Autodesk Inventor part; units mm, degrees
ref_plane "YZ Plane" through (0, 0, 0) normal (1, 0, 0) x (0, 1, 0)
ref_plane "XZ Plane" through (0, 0, 0) normal (0, 1, 0) x (-1, 0, 0)
ref_plane "XY Plane" through (0, 0, 0) normal (0, 0, 1) x (1, 0, 0)
sketch "Sketch1" plane through (0, 0, 0) normal (0, 0, 1) x (1, 0, 0)
  line L0 (0, 6) -> (0, 9)
  line L1 (0, 9) -> (10, 9)
  line L2 (10, 9) -> (10, 0)
  line L3 (10, 0) -> (0, 0)
  line L4 (0, 6) -> (5.5, 6)
  line L5 (5.5, 6) -> (7.5, 4)
  line L6 (7.5, 4) -> (7.5, 0)
  point P0 (5, 9)
  dimension "d0" = 45
  dimension "d1" = 18
  dimension "d2" = 12
  dimension "d3" = 2.5
  dimension "d4" = 10
  dimension "d5" = 2
revolve "Revolution1" add sketch "Sketch1" angle 360 about axis through (10, 0, 0) along (-1, 0, 0)
thread "Thread1"
sketch "Sketch2" plane through (10, 0, 0) normal (1, 0, 0) x (0, 0, -1)
  circle A0 centre (0, 0) radius 9
hole "Hole1" at (10, 0, 0) direction (-1, 0, 0) diameter 6 end through all
fillet "Fillet1" radius 2 1 edges at (10, -9, 0)
properties part number "14.2"
The model under review builds one solid part; all positions refer to its coordinate system, in mm. A direction names the side the tool comes from. Give positions to 0.01 mm unless a question says otherwise; leave off trailing zeros. Write each loop counter-clockwise with the first axis right and the second up, starting at its lowest first coordinate (ties: lowest second). Pieces come first, ordered by that corner, then holes. Notation, with made-up numbers: M 70,30.5 L 124,30.5 A29 cw 124,60.5 Z; hole C -37,65 d2. An arc over 180 degrees is marked long. One line per question, with ' | ' between items. Start each with the question number.
Item 1: We need section B-B on x = 1.75. Write out the cut boundary in (y, z), plus the area to 3 significant figures.
Item 2: For faces 1 (the cylindrical face through (9, 0, 3)), 2 (the flat face through (7.5, 1, -3)), list the 3-axis set-ups (+Z, -Z, +X, -X, +Y, -Y) from which the entire face can be reached by the end or side of a thin tool; tool diameter is ignored.
Item 3: Draft analysis for pull direction Z (two halves, no side actions). For faces 3 (the flat face through (10, 1, 3)), 4 (the cylindrical face through (3, -6, 0)), 5 (the cylindrical face through (4.056, -1.172, 8.923)), state which applies: released by +Z, released by -Z, zero draft, split by the parting line, or undercut.
Item 4: For pin 1 (7 mm diameter, centred on y = 0, z = 0, fed in from -X); pin 2 (1 mm diameter, centred on x = 6, y = 2, fed in from +Z); pin 3 (3 mm diameter, centred on y = 2.5, z = -3.5, fed in from -X), all flat-tipped, find the tip position at first contact; note any pin that passes through.
Item 5: We need section C-C on x = 7. Write out the cut boundary in (y, z).
Item 6: We need section A-A on y = 0. Write out the cut boundary in (x, z).
Item 7: Wall thickness on line 1 (Y direction, x = 3.2, z = 0); line 2 (Y direction, x = 8.1, z = 0): over which ranges is each line inside the solid? List them lowest first. Write a range as from..to.
Results found:
1) outline: C 0,0 d18; hole C 0,0 d12 | area: 141 mm2
2) face 1: +X, -X | face 2: -X
3) face 3: zero draft | face 4: undercut | face 5: split by the parting line
4) pin 1: stops at x = 7.5 | pin 2: stops at z = 8.87 | pin 3: stops at x = 5.7
5) outline: C 0,0 d18; hole C 0,0 d9
6) outline: M 0,-9 L 8,-9 A2 ccw 10,-7 L 10,-3 L 7.5,-3 L 7.5,-4 L 5.5,-6 L 0,-6 Z; M 0,6 L 5.5,6 L 7.5,4 L 7.5,3 L 10,3 L 10,7 A2 ccw 8,9 L 0,9 Z
7) line 1: y = -9..-6, 6..9 | line 2: y = -9..-3, 3..9
